Autodesk Inventor part; units mm, degrees
ref_plane "YZ Plane" through (0, 0, 0) normal (1, 0, 0) x (0, 1, 0)
ref_plane "XZ Plane" through (0, 0, 0) normal (0, 1, 0) x (-1, 0, 0)
ref_plane "XY Plane" through (0, 0, 0) normal (0, 0, 1) x (1, 0, 0)
sketch "Эскиз1" plane through (0, 0, 0) normal (0, 1, 0) x (-1, 0, 0)
  circle A0 centre (0, 0) radius 40
  line L0 (40, 0) -> (20, -34.641)
  line L1 (20, -34.641) -> (-20, -34.641)
  line L2 (-20, -34.641) -> (-40, 0)
  line L3 (-40, 0) -> (-20, 34.641)
  line L4 (-20, 34.641) -> (20, 34.641)
  line L5 (20, 34.641) -> (40, 0)
  dimension "d0" = 80
extrude "Выдавливание1" add sketch "Эскиз1" along normal blind 90 contours L0 L1 L2 L3 L4 L5
sketch "Эскиз3" plane through (0, 0, 0) normal (1, 0, 0) x (0, 1, 0)
  line L0 (0, 0) -> (10, 0)
  line L1 (90, 0) -> (70, 0)
  line L2 (70, 0) -> (70, -20)
  line L3 (70, -20) -> (10, 0)
  line L4 (70, 0) -> (70, 20)
  line L5 (70, 20) -> (40, 20)
  line L6 (40, 20) -> (10, 0)
extrude "Выдавливание3" cut sketch "Эскиз3" against normal mid plane 90
Can you work these out from the model? Positions are in its coordinate system, mm. A direction names the side the tool comes from. Round coordinates to 2 decimals unless told otherwise and drop trailing zeros. Write each loop counter-clockwise with the first axis right and the second up, starting at its lowest first coordinate (ties: lowest second). Pieces come first, ordered by that corner, then holes. Notation, with made-up numbers: (38, -11.75) - (51, -11.75) arc R34 cw to (51, 21.25) - close; hole circle Ø9 at (67.5, -38). An arc over 180 degrees is marked (long way). Write each question's results on one line, items separated by ' | '. Start each with the question number.
1) For pin 1 Ø8 at (x, y) = (27, 58.5) entering from +Z; pin 2 Ø5 at (x, y) = (26.5, 60) entering from -Z, each with a flat end and sliding along its axis, tell me the tip position at first contact or that it passes through.
2) Which directions (+Z, -Z, +X, -X, +Y, -Y) give clear straight access to the entire face, cutting with the end or side of a thin tool? Please do faces 1 (the flat face through (1, 70, 0)), 2 (the flat face through (-27.918, 44.37, -20.927)).
3) Suppose I cut it at D-D (y = 79). List the corners of the cut face in (x, z) for me.
4) Please list where these lines run through material, in increasing order: line 1 (Z direction, x = -24, y = 30.5); line 2 (Z direction, x = 13, y = 63.5); line 3 (X direction, y = 30, z = -20).
5) Suppose I cut it at B-B (y = 57). List the corners of the cut face in (x, z) for me.
6) Suppose I cut it at A-A (z = 7.5). List the corners of the cut face in (x, y) for me, and give its area (3 significant figures).
7) Suppose I cut it at C-C (x = 24). List the corners of the cut face in (y, z) for me, and give its area (3 significant figures).
8) We'd pull the mould along Z, two halves only. Please class faces 3 (the flat face through (1, 90, 0)), 4 (the flat face through (27.918, 44.37, 20.927)), 5 (the flat face through (0, 44, -34.641)), 6 (the flat face through (0, 55, 20)): released by +Z, released by -Z, zero draft, split by the parting line, or undercut.
Here are the results:
1) pin 1: stops at z = 29.44 | pin 2: stops at z = -27.71
2) face 1: +X, -X | face 2: -Z, -X, +Y, -Y
3) outline: (-40, 0) - (-20, -34.64) - (20, -34.64) - (40, 0) - (20, 34.64) - (-20, 34.64) - close
4) line 1: z = -27.71 to -6.83, 13.67 to 27.71 | line 2: z = -34.64 to -17.83, 20 to 34.64 | line 3: x = -28.45 to 28.45
5) outline: (-30.95, -15.67) - (-20, -34.64) - (20, -34.64) - (30.95, -15.67) - close; (-28.45, 20) - (28.45, 20) - (20, 34.64) - (-20, 34.64) - close
6) outline: (-35.67, 0) - (35.67, 0) - (35.67, 21.25) - (-35.67, 21.25) - close; (-35.67, 70) - (35.67, 70) - (35.67, 90) - (-35.67, 90) - close | area: 2,940 mm2
7) outline: (0, -27.71) - (90, -27.71) - (90, 27.71) - (0, 27.71) - close; hole (10, 0) - (70, -20) - (70, 20) - (40, 20) - close | area: 3,490 mm2
8) face 3: zero draft | face 4: released by +Z | face 5: released by -Z | face 6: undercut
